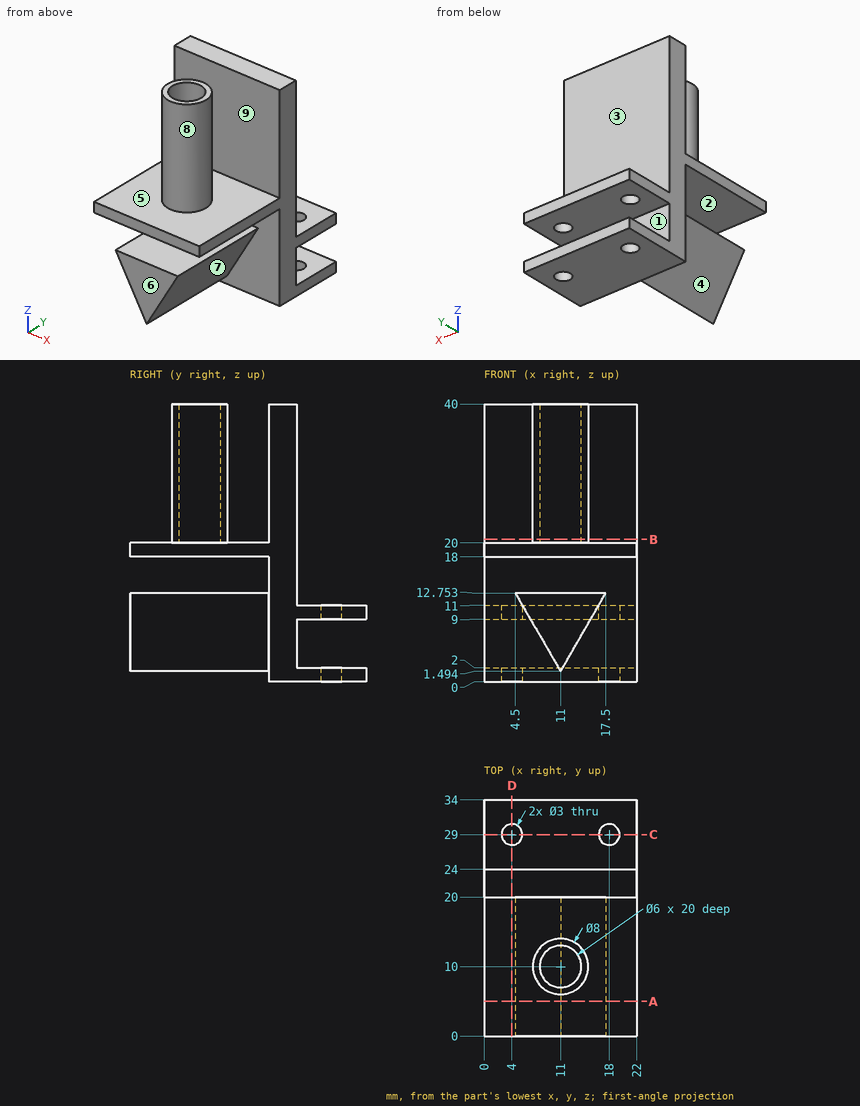
Can you work these out from the drawing? Everything is in mm from the part's minimum corner. A direction names the side the tool comes from. Coordinates: 2 decimals unless noted, no trailing zeros. Order: outer loops, then holes, each group sorted by start corner. A loop starts at its lowest first (then second) coordinate and runs counter-clockwise, first axis right, second up. Notation, with made-up numbers: M 71,-26.75 L 127,-26.75 A25 ccw 127,-5.75 Z; hole C -29.75,-32 d2. An arc over 180 degrees is marked long. Answer as CSV lines item,"result". Start each with the question number.
1. On a 3-axis mill with a long thin cutter (end or side, diameter ignored), from which of +Z, -Z, +X, -X, +Y, -Y can I reach the whole of each face in a straight line? I mean the marked faces 1, 2, 3, 4 and 5. Say none if no direction works.
2. I need wall thicknesses on line 1 (Y direction, x = 11, z = 25); line 2 (Y direction, x = 4, z = 1.3); line 3 (Z direction, x = 15.25, y = 32). Which ranges of each line are inside material? Lowest first, please. Write a range as [from, to].
3. I want a section at B-B, the plane z = 20.5. Write out the boundary of the cut face in (x, y), and give its area (3 significant figures).
4. We'd pull the mould along Y, two halves only. Please class the marked faces 6, 7, 8 and 9: released by +Y, released by -Y, zero draft, split by the parting line, or undercut.
5. I want a section at C-C, the plane y = 29. Write out the boundary of the cut face in (x, z).
6. I want a section at D-D, the plane x = 4. Write out the boundary of the cut face in (y, z), and give its area (3 significant figures).
7. For pin 1 (5 mm diameter, centred on x = 5.5, y = 31.5, fed in from +Z); pin 2 (6 mm diameter, centred on x = 14.5, z = 29, fed in from -Y); pin 3 (5 mm diameter, centred on x = 4.5, z = 30, fed in from +Y); pin 4 (1.8 mm diameter, centred on x = 18, y = 29, fed in from +Z), each with a flat end and sliding along its axis, tell me the tip position at first contact or that it passes through.
8. I want a section at A-A, the plane y = 5. Write out the boundary of the cut face in (x, z) (1 decimal), and give its area (3 significant figures).
Recorded:
1,face 1,"+X, -X, +Y"
1,face 2,"+X, -X, -Y"
1,face 3,"+Z, +X, -X, +Y"
1,face 4,"-Z, -X, -Y"
1,face 5,"+Z"
2,line 1,"y = [6, 7], [13, 14], [20, 24]"
2,line 2,"y = [20, 27.5], [30.5, 34]"
2,line 3,"z = [0, 2], [9, 11]"
3,outline,"M 0,20 L 22,20 L 22,24 L 0,24 Z; C 11,10 d8; hole C 11,10 d6"
3,area,"110 mm2"
4,face 6,"released by -Y"
4,face 7,"zero draft"
4,face 8,"undercut"
4,face 9,"undercut"
5,outline,"M 0,0 L 2.5,0 L 2.5,2 L 0,2 Z; M 0,9 L 2.5,9 L 2.5,11 L 0,11 Z; M 5.5,0 L 16.5,0 L 16.5,2 L 5.5,2 Z; M 5.5,9 L 16.5,9 L 16.5,11 L 5.5,11 Z; M 19.5,0 L 22,0 L 22,2 L 19.5,2 Z; M 19.5,9 L 22,9 L 22,11 L 19.5,11 Z"
6,outline,"M 0,18 L 20,18 L 20,0 L 27.5,0 L 27.5,2 L 24,2 L 24,9 L 27.5,9 L 27.5,11 L 24,11 L 24,40 L 20,40 L 20,20 L 0,20 Z; M 30.5,0 L 34,0 L 34,2 L 30.5,2 Z; M 30.5,9 L 34,9 L 34,11 L 30.5,11 Z"
6,area,"228 mm2"
7,pin 1,"stops at z = 11"
7,pin 2,"stops at y = 6.03"
7,pin 3,"stops at y = 24"
7,pin 4,"passes through"
8,outline,"M 0,18 L 22,18 L 22,20 L 0,20 Z; M 4.5,12.8 L 11,1.5 L 17.5,12.8 Z"
8,area,"117 mm2"
